Design review of the part built by this model. Coordinates are the model's own, in mm. A direction names the side the tool comes from. Give positions to 0.01 mm unless a question says otherwise; leave off trailing zeros. Loops run counter-clockwise (first coordinate to the right, second up) from the corner with the lowest first, then second, coordinate; pieces in that order, holes last. Notation, with made-up numbers: (18.5, 79.5) -> (52.5, 79.5) arc R22 ccw to (52.5, 95.5) -> close; hole circle Ø11 at (86, -29). An arc over 180 degrees is marked (long way). Answer as CSV lines item,"result".
from build123d import *

# Parameters (mm, degrees)
F0_W     = 38
F0_H     = 38
F1_DEPTH = 39
F2_R     = 11
F2_R_2   = 8
F3_DEPTH = 13
F4_R     = 8
F5_DEPTH = 30
F6_R     = 14.1
F7_DEPTH = 23


with BuildPart() as f1:
    # F0 (on Front) → F1 (new body)
    with BuildSketch(Plane.XZ):
        Rectangle(F0_W, F0_H)
    extrude(amount=F1_DEPTH)

    # F2 (on face) → F3 (join)
    with BuildSketch(Plane.XZ.offset(39)):
        Circle(F2_R)
        Circle(F2_R_2, mode=Mode.SUBTRACT)
    extrude(amount=F3_DEPTH)

    # F4 (on face) → F5 (cut)
    with BuildSketch(Plane.XZ.offset(39)):
        Circle(F4_R)
    extrude(amount=-F5_DEPTH, mode=Mode.SUBTRACT)

    # F6 (on face) → F7 (cut)
    with BuildSketch(Plane(origin=(-19, 0, 0), x_dir=(0, -1, 0), z_dir=(-1, 0, 0))):
        with Locations((19, 0)):
            Circle(F6_R)
    extrude(amount=-F7_DEPTH, mode=Mode.SUBTRACT)


solid = f1.part
Q1. We need section A-A, the plane z = 0. State the section outline as (x, y) points, and give its area (3 significant figures).
Filled sheet:
outline,"(-19, -39) -> (-11, -39) -> (-11, -52) -> (-8, -52) -> (-8, -33.1) -> (-19, -33.1) -> close; (-19, -4.9) -> (4, -4.9) -> (4, -9) -> (8, -9) -> (8, -52) -> (11, -52) -> (11, -39) -> (19, -39) -> (19, 0) -> (-19, 0) -> close"
area,"721 mm^2"
Q2. We need section B-B, the plane y = -19. State the section outline as (x, z) points, and give its area (3 significant figures).
Filled sheet:
outline,"(-19, -19) -> (19, -19) -> (19, 19) -> (-19, 19) -> (-19, 14.1) -> (4, 14.1) -> (4, 6.93) arc R8 cw to (4, -6.93) -> (4, -14.1) -> (-19, -14.1) -> close"
area,"756 mm^2"
Q3. We need section D-D, the plane y = -42. State the section outline as (x, z) points.
Filled sheet:
outline,"circle Ø22 at (0, 0); hole circle Ø16 at (0, 0)"
Q4. To check wall thickness, follow probe 1 along Z at (x, y) = (-8, -19); probe 2 along X at (y, z) = (-34.5, 0); probe 3 along X at (y, z) = (-28, -9). State the ranges of each line that lie inside material, in increasing order. Write a range as from..to.
Filled sheet:
probe 1,"z = -19..-14.1, 14.1..19"
probe 2,"x = -19..-8, 8..19"
probe 3,"x = 4..19"
Q5. For faces 1 (the flat face through (6, -9, 0)), 2 (the cylindrical face through (7.63, -34.98, 2.4)), 3 (the flat face through (0, -19, -19)), list the 3-axis set-ups (+Z, -Z, +X, -X, +Y, -Y) from which the entire face can be reached by the end or side of a thin tool; tool diameter is ignored.
Filled sheet:
face 1,"-X, -Y"
face 2,"-Y"
face 3,"-Z, +X, -X, +Y, -Y"
Q6. We need section C-C, the plane x = -4. State the section outline as (y, z) points.
Filled sheet:
outline,"(-52, -10.25) -> (-39, -10.25) -> (-39, -19) -> (0, -19) -> (0, 19) -> (-39, 19) -> (-39, 10.25) -> (-52, 10.25) -> (-52, 6.93) -> (-31.28, 6.93) arc R14.1 cw (long way) to (-31.28, -6.93) -> (-52, -6.93) -> close"
Q7. The part is to be moulded in two halves that separate along Y. For faces 4 (the cylindrical face through (-7.661, -4.914, 0.62)), 5 (the flat face through (4, -17.1, 7.4)), 6 (the cylindrical face through (-2.38, -45.41, -10.74)), 7 (the flat face through (-9, -39, -8)), say which applies: pulls with the +Y half, pulls with the -Y half, needs draft (parallel to the pull), parting line crosses it, or undercut.
Filled sheet:
face 4,"undercut"
face 5,"undercut"
face 6,"needs draft"
face 7,"pulls with the -Y half"
Q8. Clearance check with flat-ended pins moving along their axes: pin 1 Ø1.5 at (x, z) = (12.5, 3) entering from +Y; pin 2 Ø3 at (x, z) = (5, -1.5) entering from -Y; pin 3 Ø1 at (x, z) = (-13, 1) entering from -Y; pin 4 Ø6 at (x, y) = (0.5, -44.5) entering from -Z. State where each tip first meets the part, or that it passes through.
Filled sheet:
pin 1,"stops at y = 0"
pin 2,"stops at y = -9"
pin 3,"stops at y = -39"
pin 4,"stops at z = -11"
